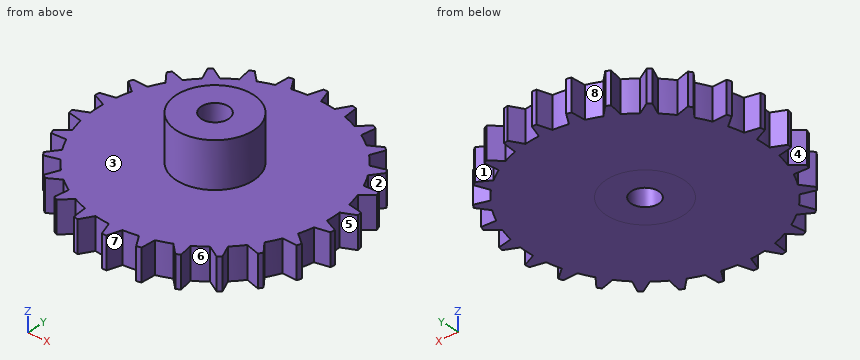
from build123d import *

# Parameters (mm, degrees)
SKETCH1_R                = 8.5
BOSS_EXTRUDE1_DEPTH      = 7
SKETCH2_R                = 8.5
SKETCH2_R_2              = 3
BOSS_EXTRUDE2_DEPTH      = 10
BOSS_EXTRUDE2_DEPTH_BACK = 7


with BuildPart() as part:
    # Sketch1 → Boss-Extrude1 (new body)
    with BuildSketch(Plane.XY):
        with BuildLine():
            Line((6.453651746, 28.272785132), (4.75543091, 25.561413828))
            ThreePointArc((4.75543091, 25.561413828), (3.133953687, 25.810430727), (1.5, 25.956694705))
            Line((1.5, 25.956694705), (0.5, 28.995689335))
            Line((0.5, 28.995689335), (-0.5, 28.995689335))
            Line((-0.5, 28.995689335), (-1.5, 25.956694705))
            ThreePointArc((-1.5, 25.956694705), (-3.133953687, 25.810430727), (-4.75543091, 25.561413828))
            Line((-4.75543091, 25.561413828), (-6.453651746, 28.272785132))
            Line((-6.453651746, 28.272785132), (-7.424593563, 28.033469468))
            Line((-7.424593563, 28.033469468), (-7.668256362, 24.843466835))
            ThreePointArc((-7.668256362, 24.843466835), (-9.219727063, 24.31042231), (-10.734493461, 23.680596491))
            Line((-10.734493461, 23.680596491), (-13.03224071, 25.906769425))
            Line((-13.03224071, 25.906769425), (-13.917696736, 25.442046253))
            Line((-13.917696736, 25.442046253), (-13.390861537, 22.286426974))
            ThreePointArc((-13.390861537, 22.286426974), (-14.769683415, 21.397580513), (-16.08970627, 20.423548961))
            Line((-16.08970627, 20.423548961), (-18.853443215, 22.035146447))
            Line((-18.853443215, 22.035146447), (-19.601953963, 21.372023789))
            Line((-19.601953963, 21.372023789), (-18.335238514, 18.434180986))
            ThreePointArc((-18.335238514, 18.434180986), (-19.461279452, 17.241189114), (-20.509843834, 15.979559002))
            Line((-20.509843834, 15.979559002), (-23.57895213, 16.882920851))
            Line((-23.57895213, 16.882920851), (-24.147016876, 16.059936985))
            Line((-24.147016876, 16.059936985), (-22.214038074, 13.510607405))
            ThreePointArc((-22.214038074, 13.510607405), (-23.021856667, 12.082802473), (-23.738023825, 10.606895158))
            Line((-23.738023825, 10.606895158), (-26.934138052, 10.749521263))
            Line((-26.934138052, 10.749521263), (-27.288742939, 9.81450502))
            Line((-27.288742939, 9.81450502), (-24.801838486, 7.80184643))
            ThreePointArc((-24.801838486, 7.80184643), (-25.244487253, 6.222207271), (-25.586636155, 4.617797121))
            Line((-25.586636155, 4.617797121), (-28.724009773, 3.991398571))
            Line((-28.724009773, 3.991398571), (-28.844546453, 2.998689697))
            Line((-28.844546453, 2.998689697), (-25.948246196, 1.639670499))
            ThreePointArc((-25.948246196, 1.639670499), (-26, 0), (-25.948246196, -1.639670499))
            Line((-25.948246196, -1.639670499), (-28.844546453, -2.998689697))
            Line((-28.844546453, -2.998689697), (-28.724009773, -3.991398571))
            Line((-28.724009773, -3.991398571), (-25.586636155, -4.617797121))
            ThreePointArc((-25.586636155, -4.617797121), (-25.244487253, -6.222207271), (-24.801838486, -7.80184643))
            Line((-24.801838486, -7.80184643), (-27.288742939, -9.81450502))
            Line((-27.288742939, -9.81450502), (-26.934138052, -10.749521263))
            Line((-26.934138052, -10.749521263), (-23.738023825, -10.606895158))
            ThreePointArc((-23.738023825, -10.606895158), (-23.021856667, -12.082802473), (-22.214038074, -13.510607405))
            Line((-22.214038074, -13.510607405), (-24.147016876, -16.059936985))
            Line((-24.147016876, -16.059936985), (-23.57895213, -16.882920851))
            Line((-23.57895213, -16.882920851), (-20.509843834, -15.979559002))
            ThreePointArc((-20.509843834, -15.979559002), (-19.461279452, -17.241189114), (-18.335238514, -18.434180986))
            Line((-18.335238514, -18.434180986), (-19.601953963, -21.372023789))
            Line((-19.601953963, -21.372023789), (-18.853443215, -22.035146447))
            Line((-18.853443215, -22.035146447), (-16.08970627, -20.423548961))
            ThreePointArc((-16.08970627, -20.423548961), (-14.769683415, -21.397580513), (-13.390861537, -22.286426974))
            Line((-13.390861537, -22.286426974), (-13.917696736, -25.442046253))
            Line((-13.917696736, -25.442046253), (-13.03224071, -25.906769425))
            Line((-13.03224071, -25.906769425), (-10.734493461, -23.680596491))
            ThreePointArc((-10.734493461, -23.680596491), (-9.219727063, -24.31042231), (-7.668256362, -24.843466835))
            Line((-7.668256362, -24.843466835), (-7.424593563, -28.033469468))
            Line((-7.424593563, -28.033469468), (-6.453651746, -28.272785132))
            Line((-6.453651746, -28.272785132), (-4.75543091, -25.561413828))
            ThreePointArc((-4.75543091, -25.561413828), (-3.133953687, -25.810430727), (-1.5, -25.956694705))
            Line((-1.5, -25.956694705), (-0.5, -28.995689335))
            Line((-0.5, -28.995689335), (0.5, -28.995689335))
            Line((0.5, -28.995689335), (1.5, -25.956694705))
            ThreePointArc((1.5, -25.956694705), (3.133953687, -25.810430727), (4.75543091, -25.561413828))
            Line((4.75543091, -25.561413828), (6.453651746, -28.272785132))
            Line((6.453651746, -28.272785132), (7.424593563, -28.033469468))
            Line((7.424593563, -28.033469468), (7.668256362, -24.843466835))
            ThreePointArc((7.668256362, -24.843466835), (9.219727063, -24.31042231), (10.734493461, -23.680596491))
            Line((10.734493461, -23.680596491), (13.03224071, -25.906769425))
            Line((13.03224071, -25.906769425), (13.917696736, -25.442046253))
            Line((13.917696736, -25.442046253), (13.390861537, -22.286426974))
            ThreePointArc((13.390861537, -22.286426974), (14.769683415, -21.397580513), (16.08970627, -20.423548961))
            Line((16.08970627, -20.423548961), (18.853443215, -22.035146447))
            Line((18.853443215, -22.035146447), (19.601953963, -21.372023789))
            Line((19.601953963, -21.372023789), (18.335238514, -18.434180986))
            ThreePointArc((18.335238514, -18.434180986), (19.461279452, -17.241189114), (20.509843834, -15.979559002))
            Line((20.509843834, -15.979559002), (23.57895213, -16.882920851))
            Line((23.57895213, -16.882920851), (24.147016876, -16.059936985))
            Line((24.147016876, -16.059936985), (22.214038074, -13.510607405))
            ThreePointArc((22.214038074, -13.510607405), (23.021856667, -12.082802473), (23.738023825, -10.606895158))
            Line((23.738023825, -10.606895158), (26.934138052, -10.749521263))
            Line((26.934138052, -10.749521263), (27.288742939, -9.81450502))
            Line((27.288742939, -9.81450502), (24.801838486, -7.80184643))
            ThreePointArc((24.801838486, -7.80184643), (25.244487253, -6.222207271), (25.586636155, -4.617797121))
            Line((25.586636155, -4.617797121), (28.724009773, -3.991398571))
            Line((28.724009773, -3.991398571), (28.844546453, -2.998689697))
            Line((28.844546453, -2.998689697), (25.948246196, -1.639670499))
            ThreePointArc((25.948246196, -1.639670499), (26, 0), (25.948246196, 1.639670499))
            Line((25.948246196, 1.639670499), (28.844546453, 2.998689697))
            Line((28.844546453, 2.998689697), (28.724009773, 3.991398571))
            Line((28.724009773, 3.991398571), (25.586636155, 4.617797121))
            ThreePointArc((25.586636155, 4.617797121), (25.244487253, 6.222207271), (24.801838486, 7.80184643))
            Line((24.801838486, 7.80184643), (27.288742939, 9.81450502))
            Line((27.288742939, 9.81450502), (26.934138052, 10.749521263))
            Line((26.934138052, 10.749521263), (23.738023825, 10.606895158))
            ThreePointArc((23.738023825, 10.606895158), (23.021856667, 12.082802473), (22.214038074, 13.510607405))
            Line((22.214038074, 13.510607405), (24.147016876, 16.059936985))
            Line((24.147016876, 16.059936985), (23.57895213, 16.882920851))
            Line((23.57895213, 16.882920851), (20.509843834, 15.979559002))
            ThreePointArc((20.509843834, 15.979559002), (19.461279452, 17.241189114), (18.335238514, 18.434180986))
            Line((18.335238514, 18.434180986), (19.601953963, 21.372023789))
            Line((19.601953963, 21.372023789), (18.853443215, 22.035146447))
            Line((18.853443215, 22.035146447), (16.08970627, 20.423548961))
            ThreePointArc((16.08970627, 20.423548961), (14.769683415, 21.397580513), (13.390861537, 22.286426974))
            Line((13.390861537, 22.286426974), (13.917696736, 25.442046253))
            Line((13.917696736, 25.442046253), (13.03224071, 25.906769425))
            Line((13.03224071, 25.906769425), (10.734493461, 23.680596491))
            ThreePointArc((10.734493461, 23.680596491), (9.219727063, 24.31042231), (7.668256362, 24.843466835))
            Line((7.668256362, 24.843466835), (7.424593563, 28.033469468))
            Line((7.424593563, 28.033469468), (6.453651746, 28.272785132))
        make_face()
        Circle(SKETCH1_R, mode=Mode.SUBTRACT)
    extrude(amount=BOSS_EXTRUDE1_DEPTH)

    # Sketch2 → Boss-Extrude2 (add, two sides)
    with BuildSketch(Plane.XY.offset(7)) as boss_extrude2_sk:
        Circle(SKETCH2_R)
        Circle(SKETCH2_R_2, mode=Mode.SUBTRACT)
    extrude(amount=BOSS_EXTRUDE2_DEPTH)
    extrude(boss_extrude2_sk.sketch, amount=-BOSS_EXTRUDE2_DEPTH_BACK)


solid = part.part
Could you check a few things on this model? Use its own coordinates, in mm. Face numbers are marked on the shaded views. A direction names the side the tool comes from. Give positions to 0.01 mm unless a question says otherwise; leave off trailing zeros. Write each loop counter-clockwise with the first axis right and the second up, starting at its lowest first coordinate (ties: lowest second). Pieces come first, ordered by that corner, then holes. Notation, with made-up numbers: (19, 80.25) - (60, 80.25) arc R18 ccw to (60, 89.25) - close; hole circle Ø9 at (78, 51). An arc over 180 degrees is marked (long way). Use CSV: the item, a comma, the result in double quotes. Start each with the question number.
Item 1: For the marked faces 5, 6, 7 and 8, which set-ups out of +Z, -Z, +X, -X, +Y, -Y let a thin tool reach every point of the face, with its end or its side?
Item 2: I'm going to push flat-ended pins straight in: pin 1 (17.5 mm diameter, centred on x = 10.5, y = 6, fed in from +Z); pin 2 (5 mm diameter, centred on x = -6, z = 3.5, fed in from +Y); pin 3 (2 mm diameter, centred on x = -4.5, z = 4, fed in from +Y); pin 4 (5 mm diameter, centred on x = 22.5, z = 7.5, fed in from -Y). Where does each tip first touch, or does it pass through?
Item 3: I want a section at A-A, the plane y = 0. Please give me the cut outline in (x, z), then the cut area to 3 significant figures.
Item 4: If I drill on line 1 along Y through (x, z) = (0, 10); line 2 along Y through (x, z) = (0, 4); line 3 along X through (y, z) = (-21.5, 4), over which ranges is the centre line in solid material (lowest first)?
Item 5: I want a section at B-B, the plane y = -23. Please give me the cut outline in (x, z).
Item 6: I want a section at C-C, the plane y = 12.5. Please give me the cut outline in (x, z).
Item 7: If we mould it in two halves opening along X, with no side actions, what happens to the marked faces 1, 2, 3 and 4? For each: pulls with the +X half, pulls with the -X half, needs draft (parallel to the pull), parting line crosses it, or undercut.
Findings:
1,face 5,"+Z, -Z, +X"
1,face 6,"+Z, -Z"
1,face 7,"+Z, -Z, -Y"
1,face 8,"+Z, -Z, +Y"
2,pin 1,"stops at z = 17"
2,pin 2,"stops at y = 28.27"
2,pin 3,"stops at y = 26.75"
2,pin 4,"stops at y = -16.88"
3,outline,"(-26, 0) - (-3, 0) - (-3, 17) - (-8.5, 17) - (-8.5, 7) - (-26, 7) - close; (3, 0) - (26, 0) - (26, 7) - (8.5, 7) - (8.5, 17) - (3, 17) - close"
3,area,"432 mm2"
4,line 1,"y = -8.5 to -3, 3 to 8.5"
4,line 2,"y = -29 to -3, 3 to 29"
4,line 3,"x = -19.46 to -17.94, -14.62 to 14.62, 17.94 to 19.46"
5,outline,"(-13.51, 0) - (13.51, 0) - (13.51, 7) - (-13.51, 7) - close"
6,outline,"(-22.8, 0) - (22.8, 0) - (22.8, 7) - (-22.8, 7) - close"
7,face 1,"undercut"
7,face 2,"pulls with the +X half"
7,face 3,"needs draft"
7,face 4,"pulls with the -X half"
